Source: CAD feature listing. Evaluate the final solid. Frame: model axes, mm. A direction names the side the tool comes from. Coordinates: 2 decimals unless noted, no trailing zeros. Loops run counter-clockwise (first coordinate to the right, second up) from the corner with the lowest first, then second, coordinate; pieces in that order, holes last. Notation, with made-up numbers: (39, 53) - (90, 53) arc R24 cw to (90, 72) - close; hole circle Ø11 at (6, -35). An arc over 180 degrees is marked (long way). Use one line per item in the form item = value. Start each with the question number.
from build123d import *

# Parameters (mm, degrees)
F0_W      = 130
F0_H      = 84
F1_DEPTH  = 25.5
F2_W      = 78.4
F2_H      = 16
F3_DEPTH  = 128
F4_W      = 115
F4_H      = 67.26
F5_DEPTH  = 25.501
F6_R      = 1.75
F7_DEPTH  = 130.001
F9_R      = 3
F10_DEPTH = 25
F11_R     = 3
F12_DEPTH = 25


with BuildPart() as f1:
    # F0 (on Top) → F1 (new body)
    with BuildSketch(Plane.XY):
        with Locations((-20.303967, 1.606347)):
            Rectangle(F0_W, F0_H)
    extrude(amount=F1_DEPTH)

    # F2 (on face) → F3 (cut)
    with BuildSketch(Plane.YZ.offset(44.696033)):
        with Locations((1.606347, 12.75)):
            Rectangle(F2_W, F2_H)
    extrude(amount=-F3_DEPTH, mode=Mode.SUBTRACT)

    # F4 (on face) → F5 (cut, through all)
    with BuildSketch(Plane.XY.offset(25.5)):
        with Locations((-12.803967, 1.606347)):
            Rectangle(F4_W, F4_H)
    extrude(amount=-F5_DEPTH, mode=Mode.SUBTRACT)

    # F6 (on face) → F7 (cut, through all)
    with BuildSketch(Plane(origin=(-85.303967, 0, 0), x_dir=(0, -1, 0), z_dir=(-1, 0, 0))):
        with Locations((0, 18.112885)):
            Circle(F6_R)
        with Locations((0, 7.387115)):
            Circle(F6_R)
        with Locations((-6.850508, 12.75)):
            Circle(F6_R)
        with Locations((6.850508, 12.75)):
            Circle(F6_R)
    extrude(amount=-F7_DEPTH, mode=Mode.SUBTRACT)

    # F9 (on face) → F10 (cut)
    with BuildSketch(Plane.YZ.offset(-83.303967)):
        with Locations((0, 18.112885)):
            Circle(F9_R)
    extrude(amount=F10_DEPTH, mode=Mode.SUBTRACT)

    # F11 (on face) → F12 (cut)
    with BuildSketch(Plane.YZ.offset(-83.303967)):
        with Locations((0, 7.387115)):
            Circle(F11_R)
    extrude(amount=F12_DEPTH, mode=Mode.SUBTRACT)


solid = f1.part
(1) Access query for faces 4 (the face through (-70.304, 1, 23)), 5 (the face through (-21, 43.606, 13)), 6 (the face through (-18, -37.594, 13)). Directions: +Z, -Z, +X, -X, +Y, -Y. A direction counts if a zero-diameter tool reaches every point of the face in a straight line with its end or side. Return the directions, or none.
(2) Cut plane D-D, the plane y = -20.5. Output: boundary loops of the cut face in (x, z), plus the area to 4 significant figures.
(3) Cut plane B-B, the plane z = 12.75. Output: boundary loops of the cut face in (x, y), plus the area to 3 significant figures.
(4) Cut plane C-C, the plane x = -62.5. Output: boundary loops of the cut face in (y, z), plus the area to 3 significant figures.
(5) Cut plane A-A, the plane y = 0. Output: boundary loops of the cut face in (x, z).
(6) Material intervals for line 1 (Z direction, x = -84, y = 0); line 2 (Y direction, x = -64.5, z = 7.5); line 3 (Z direction, x = -76, y = 6), sorted ascending.
(7) Contact query for flat-ended pins moving along their axis: pin 1 (1.4 mm diameter, centred on y = -8.5, z = 3.5, fed in from +X); pin 2 (4 mm diameter, centred on y = 9.5, z = 15, fed in from +X); pin 3 (3 mm diameter, centred on y = 0, z = 7.39, fed in from -X). Output: stop coordinate, or through.
(8) Mould query, pull axis Z, two halves, no side actions, for faces 1 (the face through (-18, 40.806, 13)), 2 (the face through (-21, -40.394, 13)), 3 (the face through (-40, 36, 25.5)). Classes: +Z half, -Z half, draft (parallel to the pull), parting line (faces both ways), or undercut.
Recorded:
q1.face_4 = +Z, -Z, +X
q1.face_5 = +Z, -Z, +X, -X, +Y
q1.face_6 = +X
q2.outline = (-85.3, 0) - (-70.3, 0) - (-70.3, 4.75) - (-83.3, 4.75) - (-83.3, 20.75) - (-70.3, 20.75) - (-70.3, 25.5) - (-85.3, 25.5) - close
q2.area = 174.5 mm²
q3.outline = (-85.3, -40.39) - (44.7, -40.39) - (44.7, -37.59) - (-83.3, -37.59) - (-83.3, -8.6) - (-85.3, -8.6) - close; (-85.3, -5.1) - (-83.3, -5.1) - (-83.3, 5.1) - (-85.3, 5.1) - close; (-85.3, 8.6) - (-83.3, 8.6) - (-83.3, 40.81) - (44.7, 40.81) - (44.7, 43.61) - (-85.3, 43.61) - close
q3.area = 871 mm²
q4.outline = (-40.39, 0) - (-32.02, 0) - (-32.02, 4.75) - (-37.59, 4.75) - (-37.59, 20.75) - (-32.02, 20.75) - (-32.02, 25.5) - (-40.39, 25.5) - close; (35.24, 0) - (43.61, 0) - (43.61, 25.5) - (35.24, 25.5) - (35.24, 20.75) - (40.81, 20.75) - (40.81, 4.75) - (35.24, 4.75) - close
q4.area = 249 mm²
q5.outline = (-85.3, 0) - (-70.3, 0) - (-70.3, 4.39) - (-83.3, 4.39) - (-83.3, 5.64) - (-85.3, 5.64) - close; (-85.3, 9.14) - (-83.3, 9.14) - (-83.3, 16.36) - (-85.3, 16.36) - close; (-85.3, 19.86) - (-83.3, 19.86) - (-83.3, 21.11) - (-70.3, 21.11) - (-70.3, 25.5) - (-85.3, 25.5) - close
q6.line_1 = 0 to 5.64, 9.14 to 16.36, 19.86 to 25.5
q6.line_2 = -40.39 to -37.59, 40.81 to 43.61
q6.line_3 = 0 to 4.75, 20.75 to 25.5
q7.pin_1 = -70.3
q7.pin_2 = -83.3
q7.pin_3 = through
q8.face_1 = undercut
q8.face_2 = draft
q8.face_3 = +Z half
